```python
from build123d import *

# Parameters (mm, degrees)
CUT_EXTRUDE_START   = -18
CUT_EXTRUDE_1_DEPTH = 18
FILLET_1_R          = 1.5


with BuildPart() as part:
    # Эскиз1 → Повернуть1 (revolve)
    with BuildSketch(Plane.XY, mode=Mode.PRIVATE) as revolve_1_sk:
        Polygon((0, 11.5), (0, 13.823673019), (1, 14), (19, 14), (20, 13.823673019), (20, 11.5), (19.5, 11), (0.5, 11), align=None)
    revolve(revolve_1_sk.sketch.rotate(Axis((-7.002814628, 0, 0), (1, 0, 0)), 90), axis=Axis((-7.002814628, 0, 0), (1, 0, 0)))

    # Эскиз2 → Вырез-Вытянуть1 (cut)
    with BuildSketch(Plane(origin=(20, 0, 0), x_dir=(0, 0, -1), z_dir=(1, 0, 0)).offset(CUT_EXTRUDE_START)):
        with BuildLine():
            ThreePointArc((-1.810386699, -10.85), (0, -11), (1.810386699, -10.85))
            ThreePointArc((1.810386699, -10.85), (0, -12), (-1.810386699, -10.85))
        make_face()
        with BuildLine():
            ThreePointArc((-1.810386699, 10.85), (0, 12), (1.810386699, 10.85))
            ThreePointArc((1.810386699, 10.85), (0, 11), (-1.810386699, 10.85))
        make_face()
    extrude(amount=CUT_EXTRUDE_1_DEPTH, mode=Mode.SUBTRACT)

    # Скругление1
    # the kernel refuses this fillet: 1.5 mm, written as the material it adds along each edge
    with BuildSketch(Plane(origin=(2, 10, 0), x_dir=(0, -0.9911428491773114, 0.132800047156171), z_dir=(0, -0.132800047156171, -0.9911428491773114))) as fillet_1_piece_1_section:
        with BuildLine():
            CenterArc((2 - FILLET_1_R, -FILLET_1_R), FILLET_1_R, 0, 90)
            Line((2, -FILLET_1_R), (2, 0))
            Line((2, 0), (2 - FILLET_1_R, 0))
        make_face()
    fillet_1_piece_1 = revolve(axis=Axis((2, 10, 0), (-1, 0, 0)), revolution_arc=344.737147097, mode=Mode.PRIVATE)
    fillet_1_piece_1 = fillet_1_piece_1 - Plane(origin=(2.626804304, 0, 0), x_dir=(0, 0, 1), z_dir=(-1, 0, 0)) * Cylinder(11, 8, mode=Mode.PRIVATE)
    add(fillet_1_piece_1)
    with BuildSketch(Plane(origin=(2, -10, 0), x_dir=(0, 0.9911428491773114, -0.132800047156171), z_dir=(0, 0.132800047156171, 0.9911428491773114))) as fillet_1_piece_2_section:
        with BuildLine():
            CenterArc((2 - FILLET_1_R, -FILLET_1_R), FILLET_1_R, 0, 90)
            Line((2, -FILLET_1_R), (2, 0))
            Line((2, 0), (2 - FILLET_1_R, 0))
        make_face()
    fillet_1_piece_2 = revolve(axis=Axis((2, -10, 0), (-1, 0, 0)), revolution_arc=344.737147097, mode=Mode.PRIVATE)
    fillet_1_piece_2 = fillet_1_piece_2 - Plane(origin=(2.626804304, 0, 0), x_dir=(0, 0, 1), z_dir=(-1, 0, 0)) * Cylinder(11, 8, mode=Mode.PRIVATE)
    add(fillet_1_piece_2)


solid = part.part
```
Geometry check sheet. Reference: the model listing, model coordinates, mm. A direction names the side the tool comes from. Round coordinates to 2 decimals unless told otherwise and drop trailing zeros. Loops run counter-clockwise (first coordinate to the right, second up) from the corner with the lowest first, then second, coordinate; pieces in that order, holes last. Notation, with made-up numbers: (51.25, 1) -> (74.25, 1) arc R25 cw to (74.25, 28) -> close; hole circle Ø1 at (-16, -6.75). An arc over 180 degrees is marked (long way). Use a Markdown table: item, result.
(1) Sectioned sample at B-B (x = 11.5). Enter the section's corners in (y, z).
Calculated:
| item | result |
|---|---|
| outline | circle Ø28 at (0, 0); hole (-10.85, -1.81) arc R11 ccw to (10.85, -1.81) arc R2 ccw to (10.85, 1.81) arc R11 ccw to (-10.85, 1.81) arc R2 ccw to start |
(2) Mould release check, pull along Z, two halves, no side actions. Record for faces 3 (the conical face through (19.635, 0.226, 11.133)), 4 (the conical face through (19.635, -0.226, -11.133)), 5 (the flat face through (20, 3, -11.3)), 6 (the cylindrical face through (10.1, 12.4, 6.5)): released by +Z, released by -Z, zero draft, split by the parting line, or undercut.
Calculated:
| item | result |
|---|---|
| face 3 | undercut |
| face 4 | undercut |
| face 5 | zero draft |
| face 6 | split by the parting line |
(3) Set-up check for faces 1 (the cylindrical face through (12, -12, 0)), 2 (the flat face through (0, 3, 11.3)): record each of +Z, -Z, +X, -X, +Y, -Y from which the full face is reachable in a straight line by a thin tool's end or side.
Calculated:
| item | result |
|---|---|
| face 1 | +X |
| face 2 | +Z, -Z, -X, +Y, -Y |
(4) Go/stop test with flat-tipped pins: P1, Ø5, axis at x = 2.5, y = -9, coming from the -Z side; P2, Ø6, axis at x = 2.5, y = -5, coming from the +Z side; P3, Ø8, axis at y = -7.5, z = 8, coming from the +X side; P4, Ø2, axis at x = 4, z = 4.5, coming from the +Y side. Record where each tip stops, or that it passes through.
Calculated:
| item | result |
|---|---|
| P1 | z = -12.4 |
| P2 | z = 13.86 |
| P3 | x = 20 |
| P4 | y = 13.56 |
(5) Scan lines: probe 1 along Y at (x, z) = (4.75, 0); probe 2 along Z at (x, y) = (13.5, 3.5); probe 3 along Z at (x, y) = (16.5, -1.75). Record each from-to range of solid material in increasing order.
Calculated:
| item | result |
|---|---|
| probe 1 | -14 to -12, 12 to 14 |
| probe 2 | -13.56 to -10.43, 10.43 to 13.56 |
| probe 3 | -13.89 to -10.86, 10.86 to 13.89 |
(6) Sectioned sample at A-A (y = 0). Enter the section's corners in (x, z), then the cut area to 3 significant figures.
Calculated:
| item | result |
|---|---|
| outline | (0, -13.82) -> (1, -14) -> (19, -14) -> (20, -13.82) -> (20, -11.5) -> (19.5, -11) -> (0.5, -11) -> (0, -11.5) -> close; (0, 11.5) -> (0.5, 11) -> (19.5, 11) -> (20, 11.5) -> (20, 13.82) -> (19, 14) -> (1, 14) -> (0, 13.82) -> close |
| area | 119 mm² |
